from build123d import *

# Parameters (mm, degrees)
CORTAR_EXTRUIR1_DEPTH = 2


with BuildPart() as part:
    # Croquis1 → Revolución1 (revolve)
    with BuildSketch(Plane.XY, mode=Mode.PRIVATE) as revoluci_n1_sk:
        Polygon((0, 0), (-1.25, 0), (-1.25, 8), (-2.2, 8), (-2.2, 10.5), (-0.840646635, 10.5), (-0.840646635, 8.822225361), (0, 8.822225361), align=None)
    revolve(revoluci_n1_sk.sketch.rotate(Axis((0, 8.822225361, 0), (0, -1, 0)), 270), axis=Axis((0, 8.822225361, 0), (0, -1, 0)))

    # Croquis2 → Cortar-Extruir1 (cut)
    with BuildSketch(Plane(origin=(0, 10.5, 0), x_dir=(1, 0, 0), z_dir=(0, 1, 0))):
        Polygon((0.875027781, 0.753431958), (-0.214977325, 1.134512267), (-1.090005106, 0.381080309), (-0.875027781, -0.753431958), (0.214977325, -1.134512267), (1.090005106, -0.381080309), align=None)
    extrude(amount=-CORTAR_EXTRUIR1_DEPTH, mode=Mode.SUBTRACT)


solid = part.part
Can you work these out from the model? Positions are in its coordinate system, mm. A direction names the side the tool comes from. Round coordinates to 2 decimals unless told otherwise and drop trailing zeros. Loops run counter-clockwise (first coordinate to the right, second up) from the corner with the lowest first, then second, coordinate; pieces in that order, holes last. Notation, with made-up numbers: (-2, 81) - (45, 81) arc R24 ccw to (45, 108) - close; hole circle Ø5 at (21.25, 10.25). An arc over 180 degrees is marked (long way). Write item = value, one per line. Start each with the question number.
(1) If we section it at B-B (z = 0): Please give me the cut outline in (x, y).
(2) If we mould it in two halves opening along X, with no side actions, what happens to faces 1 (the face through (0.34, 9.51, -0.94)), 2 (the face through (0, 0, 0)), 3 (the face through (-2.18, 9.27, -0.29))? For each: released by +X, released by -X, zero draft, split by the parting line, or undercut.
(3) If we section it at D-D (y = 5): Please give me the cut outline in (x, z).
(4) For P1, Ø2, axis at x = 0, z = 1, coming from the +Y side, with a flat end and sliding along its axis, tell me the tip position at first contact or that it passes through.
(5) For faces 4 (the face through (1.22, 4.06, -0.27)), 5 (the face through (-1, 10.5, 1)), 6 (the face through (0, 8.5, 0)), which set-ups out of +Z, -Z, +X, -X, +Y, -Y let a thin tool reach every point of the face, with its end or its side?
(6) If I drill on probe 1 along Z at (x, y) = (0.35, 9.25); probe 2 along Y at (x, z) = (0.85, -1.65); probe 3 along Z at (x, y) = (0.5, 9.5), over which ranges is the centre line in solid material (lowest first)? Write a range as [from, to].
(7) If we section it at C-C (x = 0): Please give me the cut outline in (y, z).
(8) If we section it at A-A (y = 9): Please give me the cut outline in (x, z), and give its area (3 significant figures).
Ans:
q1.outline = (-2.2, 8) - (-1.25, 8) - (-1.25, 0) - (1.25, 0) - (1.25, 8) - (2.2, 8) - (2.2, 10.5) - (1.02, 10.5) - (1.02, 8.5) - (-1.02, 8.5) - (-1.02, 10.5) - (-2.2, 10.5) - close
q2.face_1 = undercut
q2.face_2 = zero draft
q2.face_3 = split by the parting line
q3.outline = circle Ø2.5 at (0, 0)
q4.P1 = 10.5
q5.face_4 = -Y
q5.face_5 = +Z, -Z, +X, -X, +Y
q5.face_6 = +Y
q6.probe_1 = [-2.17, -0.94], [1.02, 2.17]
q6.probe_2 = [8, 10.5]
q6.probe_3 = [-2.14, -0.88], [0.89, 2.14]
q7.outline = (0, -1.25) - (8, -1.25) - (8, -2.2) - (10.5, -2.2) - (10.5, -1.06) - (8.5, -1.06) - (8.5, 1.06) - (10.5, 1.06) - (10.5, 2.2) - (8, 2.2) - (8, 1.25) - (0, 1.25) - close
q8.outline = circle Ø4.4 at (0, 0); hole (-1.09, -0.38) - (-0.21, -1.13) - (0.88, -0.75) - (1.09, 0.38) - (0.21, 1.13) - (-0.88, 0.75) - close
q8.area = 11.7 mm²
